Verification items for this drawing (mm, ordinates from the low corner). A direction names the side the tool comes from. Coordinates: 2 decimals unless noted, no trailing zeros. Order: outer loops, then holes, each group sorted by start corner. A loop starts at its lowest first (then second) coordinate and runs counter-clockwise, first axis right, second up. Notation, with made-up numbers: (-25, -11.75) -> (-12, -11.75) arc R10 cw to (-12, 6.25) -> close; hole circle Ø7 at (-26, 25). An arc over 180 degrees is marked (long way). Write each question's results on one line, items separated by ' | '. Start each with the question number.
(1) Cross-section at C-C on z = 13.5. Enter the section's corners in (x, y), and give its area (3 significant figures).
(2) Thickness scan on probe 1 along X at (y, z) = (14.25, 13.5); probe 2 along X at (y, z) = (4.25, 13.5); probe 3 along Y at (x, z) = (1.5, 18.75). Record the ranges inside material, lowest first. Write a range as [from, to].
(3) Set-up check for the marked faces 1, 2, 3, 4 and 5: record each of +Z, -Z, +X, -X, +Y, -Y from which the full face is reachable in a straight line by a thin tool's end or side.
(4) Cross-section at D-D on z = 7. Enter the section's corners in (x, y).
(5) Go/stop test with flat-tipped pins: pin 1 (1.5 mm diameter, centred on x = 5.5, z = 3.5, fed in from +Y); pin 2 (1.5 mm diameter, centred on x = 1, z = 4, fed in from +Y); pin 3 (10 mm diameter, centred on y = 15, z = 11, fed in from -X); pin 4 (1 mm diameter, centred on y = 11.5, z = 18, fed in from +X). Record where each tip stops, or that it passes through.
(6) Cross-section at B-B on y = 5. Enter the section's corners in (x, z), and give its area (3 significant figures).
(7) Cross-section at A-A on x = 3.5. Enter the section's corners in (y, z), and give its area (3 significant figures).
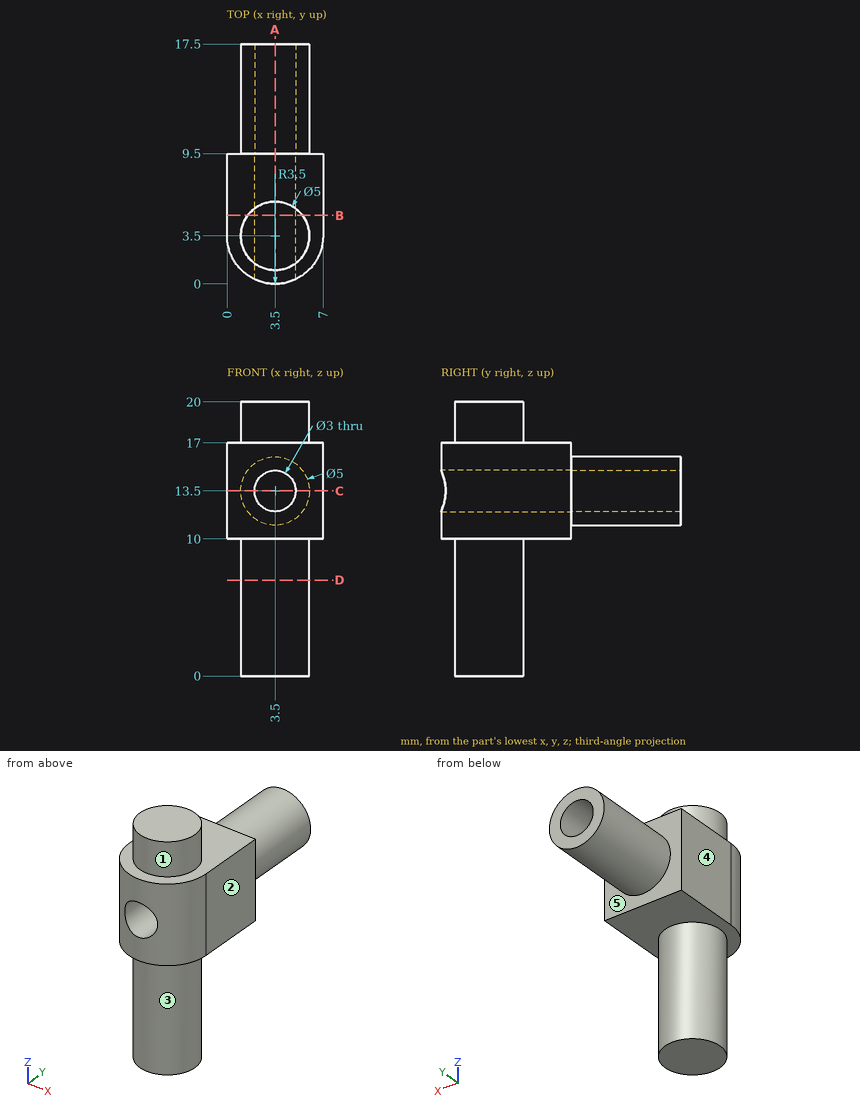
Results are:
1) outline: (0, 3.5) arc R3.5 ccw to (2, 0.34) -> (2, 17.5) -> (1, 17.5) -> (1, 9.5) -> (0, 9.5) -> close; (5, 0.34) arc R3.5 ccw to (7, 3.5) -> (7, 9.5) -> (6, 9.5) -> (6, 17.5) -> (5, 17.5) -> close | area: 49.1 mm2
2) probe 1: x = [1, 2], [5, 6] | probe 2: x = [0, 2], [5, 7] | probe 3: y = [2, 5]
3) face 1: +Z | face 2: +Z, -Z, +X, +Y, -Y | face 3: -Z | face 4: +Z, -Z, -X, +Y, -Y | face 5: +Y
4) outline: circle Ø5 at (3.5, 3.5)
5) pin 1: stops at y = 5.67 | pin 2: stops at y = 5.29 | pin 3: stops at x = 1 | pin 4: passes through
6) outline: (0, 10) -> (1.5, 10) -> (1.5, 0) -> (5.5, 0) -> (5.5, 10) -> (7, 10) -> (7, 17) -> (5.5, 17) -> (5.5, 20) -> (1.5, 20) -> (1.5, 17) -> (0, 17) -> close; hole circle Ø3 at (3.5, 13.5) | area: 93.9 mm2
7) outline: (0, 10) -> (1, 10) -> (1, 0) -> (6, 0) -> (6, 10) -> (9.5, 10) -> (9.5, 11) -> (17.5, 11) -> (17.5, 12) -> (0, 12) -> close; (0, 15) -> (17.5, 15) -> (17.5, 16) -> (9.5, 16) -> (9.5, 17) -> (6, 17) -> (6, 20) -> (1, 20) -> (1, 17) -> (0, 17) -> close | area: 119 mm2
